```python
from build123d import *

# Parameters (mm, degrees)
F1_DEPTH = 12
F2_W     = 5.9
F2_H     = 12.8
F3_DEPTH = 6.5
F4_W     = 9.5
F4_H     = 3
F5_DEPTH = 12.001
F6_R     = 3
F8_D     = 3.7973
F8_DEPTH = 13.175
F8_TIP   = 1.1408240143


with BuildPart() as f1:
    # F0 (on Top) → F1 (new body)
    with BuildSketch(Plane.XY):
        Polygon((0, 25), (-11.3, 25), (-11.3, 0), (-1.3, 0), (-1.3, 20), (0, 20), align=None)
        Polygon((15, 25), (0, 25), (0, 20), (0, 0), (15, 0), align=None)
    extrude(amount=F1_DEPTH)

    # F2 (on face) → F3 (cut)
    with BuildSketch(Plane.XY.offset(12)):
        with Locations((8.45, 10.4)):
            Rectangle(F2_W, F2_H)
    extrude(amount=-F3_DEPTH, mode=Mode.SUBTRACT)

    # F4 (on face) → F5 (cut, through all)
    with BuildSketch(Plane.XY.offset(12)):
        with Locations((10.25, 5.5)):
            Rectangle(F4_W, F4_H)
        with Locations((10.25, 10.4)):
            Rectangle(F4_W, F4_H)
        with Locations((10.25, 15.3)):
            Rectangle(F4_W, F4_H)
    extrude(amount=-F5_DEPTH, mode=Mode.SUBTRACT)

    # F6
    f6_edges = [f1.edges().sort_by_distance(p)[0] for p in [
        (-1.3, 0, 6),
        (0, 0, 6),
    ]]
    fillet(f6_edges, radius=F6_R)

    # F8
    with Locations(Plane(origin=(-11.3, 0, 0), x_dir=(0, -1, 0), z_dir=(-1, 0, 0))):
        with Locations((-7.8025250696, 6)):
            Hole(F8_D / 2, depth=F8_DEPTH)
            with Locations((0, 0, -(F8_DEPTH + F8_TIP / 2))):  # 118° drill point
                Cone(0, F8_D / 2, F8_TIP, mode=Mode.SUBTRACT)


solid = f1.part
```
CAD build for the part. Positions are in the model's coordinates, mm. A direction names the side the tool comes from. Round coordinates to 2 decimals unless told otherwise and drop trailing zeros. Order: outer loops, then holes, each group sorted by start corner. A loop starts at its lowest first (then second) coordinate and runs counter-clockwise, first axis right, second up.
Q1. Two-plate mould, pull along X, no slides. Class faces 1 (the flat face through (5.5, 10, 6)), 2 (the flat face through (15, 2, 6)), 3 (the flat face through (10, 4, 6)): pulls with the +X half, pulls with the -X half, needs draft (parallel to the pull), parting line crosses it, or undercut.
Q2. Slice it at C-C (z = 3.5). Write the cut outline in (x, y).
Q3. Which spindle directions (+Z, -Z, +X, -X, +Y, -Y) get a long thin tool onto all of the face, cutting with end or side? Do faces 4 (the flat face through (-1, 20, 6)), 5 (the flat face through (11, 11.9, 5)), 6 (the flat face through (11.4, 8, 9)). Say none if no direction does.
Q4. Slice it at B-B (y = 17.5). Write the cut outline in (x, z).
Q5. Slice it at D-D (x = -7.5). Write the cut outline in (y, z), and give its area (3 significant figures).
Q6. Wall check: L1, parallel to X at y = 12, z = 10.5; L2, parallel to X at y = 19.5, z = 9.75; L3, parallel to X at y = 11, z = 6.75. Give the ranges that are in metal, low to high.
Q7. Slice it at A-A (x = 12.25). Write the cut outline in (y, z).
Q8. Drop flat-ended pins along their axis: pin 1 (1 mm diameter, centred on y = 14.5, z = 3, fed in from +X); pin 2 (1 mm diameter, centred on x = 8.5, y = 8, fed in from +Z); pin 3 (0.6 mm diameter, centred on y = 8, z = 7.5, fed in from -X). Give the stop position or say it passes through.
Results below:
1. face 1: undercut
1. face 2: pulls with the +X half
1. face 3: needs draft
2. outline: (-11.3, 0) - (-4.3, 0) arc R3 ccw to (-1.3, 3) - (-1.3, 20) - (0, 20) - (0, 3) arc R3 ccw to (3, 0) - (15, 0) - (15, 4) - (5.5, 4) - (5.5, 7) - (15, 7) - (15, 8.9) - (5.5, 8.9) - (5.5, 11.9) - (15, 11.9) - (15, 13.8) - (5.5, 13.8) - (5.5, 16.8) - (15, 16.8) - (15, 25) - (-11.3, 25) - close
3. face 4: +Z, -Z, -Y
3. face 5: +Z, -Z, +X
3. face 6: +Z
4. outline: (-11.3, 0) - (-1.3, 0) - (-1.3, 12) - (-11.3, 12) - close; (0, 0) - (15, 0) - (15, 12) - (0, 12) - close
5. outline: (0, 0) - (25, 0) - (25, 12) - (0, 12) - close; hole circle Ø3.8 at (7.8, 6)
5. area: 289 mm2
6. L1: x = -11.3 to -1.3, 0 to 5.5, 11.4 to 15
6. L2: x = -11.3 to -1.3, 0 to 15
6. L3: x = -11.3 to -1.3, 0 to 5.5
7. outline: (0, 0) - (4, 0) - (4, 12) - (0, 12) - close; (7, 0) - (8.9, 0) - (8.9, 12) - (7, 12) - close; (11.9, 0) - (13.8, 0) - (13.8, 12) - (11.9, 12) - close; (16.8, 0) - (25, 0) - (25, 12) - (16.8, 12) - close
8. pin 1: stops at x = 5.5
8. pin 2: stops at z = 5.5
8. pin 3: stops at x = 1.93
